Design review of the part built by this model. Coordinates are the model's own, in mm. A direction names the side the tool comes from. Coordinates: 2 decimals unless noted, no trailing zeros. Write each loop counter-clockwise with the first axis right and the second up, starting at its lowest first coordinate (ties: lowest second). Pieces come first, ordered by that corner, then holes.
Q1. Take a section at A-A, the plane y = 314.5. Write out the cut boundary in (x, z) (3 decimals), plus the area to 3 significant figures.
Q2. For pin 1 Ø9 at (x, y) = (145.21, 313.63) entering from +Z; pin 2 Ø4.5 at (y, z) = (314, -1958.5) entering from +X; pin 3 Ø1.5 at (y, z) = (313.5, -1976.5) entering from -X; pin 4 Ø4.5 at (x, y) = (79.91, 313.63) entering from +Z, all flat-tipped, find the tip position at first contact; note any pin that passes through.
Q3. For faces 4 (the flat face through (122.829, 314, -1961)), 5 (the flat face through (74.829, 314, -1942)), 6 (the flat face through (140, 314, -1978.071)), list the 3-axis set-ups (+Z, -Z, +X, -X, +Y, -Y) from which the entire face can be reached by the end or side of a thin tool; tool diameter is ignored.
Q4. Take a section at D-D, the plane x = 131.5. Write out the cut boundary in (y, z).
Q5. Take a section at C-C, the plane z = -1957. Write out the cut boundary in (x, y), plus the area to 3 significant figures.
Q6. The part is to be moulded in two halves that separate along Y. For faces 1 (the cylindrical face through (81.275, 315.77, -1941.724)), 2 (the flat face through (125, 306.128, -1958)), 3 (the flat face through (98, 314, -1943.333)), say which applies: released by +Y, released by -Y, zero draft, split by the parting line, or undercut.
Q7. Take a section at B-B, the plane y = 308. Write out the cut boundary in (x, z) (3 decimals).
Q8. For L1, parallel to Z at x = 110, y = 318.25; L2, parallel to X at y = 315.75, z = -1968; L3, parallel to Z at x = 142, y = 311, list the stretches that pass through material, from the lowest coordinate up.
from build123d import *

# Parameters (mm, degrees)
SKETCH1_W                    = 48
SKETCH1_H                    = 15
BASE_FLANGE1_DEPTH           = 3.175
EDGE_FLANGE1_STRIP_W         = 14.7
EDGE_FLANGE1_STRIP_H         = 3.175
EDGE_FLANGE1_STRIP_CUT_DEPTH = 15
EDGE_FLANGE1_DEPTH           = 15
EDGE_FLANGE2_STRIP_W         = 14.7
EDGE_FLANGE2_STRIP_H         = 3.175
EDGE_FLANGE2_STRIP_CUT_DEPTH = 15
EDGE_FLANGE2_DEPTH           = 15
FILLET1_R                    = 3
SKETCH18_R                   = 2.54
CUT_EXTRUDE2_DEPTH           = 359.005866467
SKETCH19_R                   = 4
CUT_EXTRUDE3_DEPTH           = 358.655386406
M3_CLEARANCE_HOLE1_D         = 3.4


# Sheet-metal steps are written as plain solids
with BuildPart() as part:
    # Sketch1 → Base-Flange1 (new body)
    with BuildSketch(Plane.XY.offset(-1943.333434301)):
        with Locations((98.829284585, 313.628054742)):
            Rectangle(SKETCH1_W, SKETCH1_H)
    extrude(amount=BASE_FLANGE1_DEPTH)

    # Edge-Flange1 strip (across the edge) → Edge-Flange1 strip cut (cut)
    with BuildSketch(Plane(origin=(122.829284585, 321.128054742, -1943.333434301), x_dir=(-1, 0, 0), z_dir=(0, -1, 0))):
        with Locations((-6.35, -1.5875)):
            Rectangle(EDGE_FLANGE1_STRIP_W, EDGE_FLANGE1_STRIP_H)
    extrude(amount=EDGE_FLANGE1_STRIP_CUT_DEPTH, mode=Mode.SUBTRACT)

    # Edge-Flange1 section (across the edge) → Edge-Flange1 (add)
    with BuildSketch(Plane(origin=(122.829284585, 321.128054742, -1943.333434301), x_dir=(-1, 0, 0), z_dir=(0, -1, 0))):
        with BuildLine():
            Line((-3.175, 1), (-3.175, 34.7375))
            Line((-3.175, 34.7375), (0, 34.7375))
            Line((0, 34.7375), (0, 1))
            ThreePointArc((0, 1), (0.292893219, 0.292893219), (1, 0))
            Line((1, 0), (1, -3.175))
            ThreePointArc((1, -3.175), (-1.952170811, -1.952170811), (-3.175, 1))
        make_face()
    extrude(amount=EDGE_FLANGE1_DEPTH)

    # Edge-Flange2 strip (across the edge) → Edge-Flange2 strip cut (cut)
    with BuildSketch(Plane(origin=(126.004284585, 306.128054742, -1978.070934301), x_dir=(0, 0, 1), z_dir=(0, 1, 0))):
        with Locations((-6.35, -1.5875)):
            Rectangle(EDGE_FLANGE2_STRIP_W, EDGE_FLANGE2_STRIP_H)
    extrude(amount=EDGE_FLANGE2_STRIP_CUT_DEPTH, mode=Mode.SUBTRACT)

    # Edge-Flange2 section (across the edge) → Edge-Flange2 (add)
    with BuildSketch(Plane(origin=(126.004284585, 306.128054742, -1978.070934301), x_dir=(0, 0, 1), z_dir=(0, 1, 0))):
        with BuildLine():
            Line((-3.175, 1), (-3.175, 26.825))
            Line((-3.175, 26.825), (0, 26.825))
            Line((0, 26.825), (0, 1))
            ThreePointArc((0, 1), (0.292893219, 0.292893219), (1, 0))
            Line((1, 0), (1, -3.175))
            ThreePointArc((1, -3.175), (-1.952170811, -1.952170811), (-3.175, 1))
        make_face()
    extrude(amount=EDGE_FLANGE2_DEPTH)

    # Fillet1
    fillet1_edges = [part.edges().sort_by_distance(p)[0] for p in [
        (152.829284585, 306.128054742, -1979.658434301),
        (152.829284585, 321.128054742, -1979.658434301),
        (74.829284585, 306.128054742, -1941.745934301),
        (74.829284585, 321.128054742, -1941.745934301),
    ]]
    fillet(fillet1_edges, radius=FILLET1_R)

    # Sketch18 → Cut-Extrude2 (cut, through all)
    with BuildSketch(Plane.XY.offset(-1940.158434301)):
        with Locations((79.909284585, 313.628054742)):
            Circle(SKETCH18_R)
    extrude(amount=-CUT_EXTRUDE2_DEPTH, mode=Mode.SUBTRACT)

    # Sketch19 → Cut-Extrude3 (cut, through all)
    with BuildSketch(Plane.XY.offset(-1978.070934301)):
        with Locations((145.209284585, 313.628054742)):
            Circle(SKETCH19_R)
    extrude(amount=-CUT_EXTRUDE3_DEPTH, mode=Mode.SUBTRACT)

    # M3 Clearance Hole1 (through all)
    with Locations(Plane.XY.offset(-1940.158434301)):
        with Locations((117.404284585, 313.537425755)):
            Hole(M3_CLEARANCE_HOLE1_D / 2)


solid = part.part
Responses:
1. outline: (74.829, -1943.333) - (77.524, -1943.333) - (77.524, -1940.158) - (74.829, -1940.158) - close; (82.295, -1943.333) - (116.003, -1943.333) - (116.003, -1940.158) - (82.295, -1940.158) - close; (118.806, -1943.333) - (121.829, -1943.333) arc R1 cw to (122.829, -1944.333) - (122.829, -1977.071) arc R4.175 ccw to (127.004, -1981.246) - (141.305, -1981.246) - (141.305, -1978.071) - (127.004, -1978.071) arc R1 cw to (126.004, -1977.071) - (126.004, -1944.333) arc R4.175 ccw to (121.829, -1940.158) - (118.806, -1940.158) - close; (149.113, -1981.246) - (152.829, -1981.246) - (152.829, -1978.071) - (149.113, -1978.071) - close
1. area: 312 mm2
2. pin 1: stops at z = -1978.07
2. pin 2: stops at x = 126
2. pin 3: stops at x = 122.83
2. pin 4: passes through
3. face 4: -Z, -X, +Y, -Y
3. face 5: +Z, -Z, -X, +Y, -Y
3. face 6: +Z, +X, +Y, -Y
4. outline: (306.13, -1981.25) - (321.13, -1981.25) - (321.13, -1978.07) - (306.13, -1978.07) - close
5. outline: (122.83, 306.13) - (126, 306.13) - (126, 321.13) - (122.83, 321.13) - close
5. area: 47.6 mm2
6. face 1: undercut
6. face 2: released by -Y
6. face 3: zero draft
7. outline: (75.049, -1943.333) - (121.829, -1943.333) arc R1 cw to (122.829, -1944.333) - (122.829, -1977.071) arc R4.175 ccw to (127.004, -1981.246) - (152.609, -1981.246) - (152.609, -1978.071) - (127.004, -1978.071) arc R1 cw to (126.004, -1977.071) - (126.004, -1944.333) arc R4.175 ccw to (121.829, -1940.158) - (75.049, -1940.158) - close
8. L1: z = -1943.33 to -1940.16
8. L2: x = 122.83 to 126
8. L3: z = -1981.25 to -1978.07
